Model file for the job. Use its own axes, mm. Round coordinates to 2 decimals unless told otherwise and drop trailing zeros. Order: outer loops, then holes, each group sorted by start corner. A loop starts at its lowest first (then second) coordinate and runs counter-clockwise, first axis right, second up. Notation, with made-up numbers: (43, -11) -> (89, -11) arc R13 ccw to (89, -1) -> close; hole circle Ø7 at (5, 34). An arc over 180 degrees is marked (long way). Put each result on its own line as item: value. Start each with the question number.
Q1. Probe L1, parallel to X at y = 9, z = 1.5; L2, parallel to Y at x = -11, z = 0.75 (3 decimals); L3, parallel to Y at x = 26, z = 4 (3 decimals). List the from-to ranges inside material, lowest first.
Q2. Flat gauge pins, fed straight in: P1, Ø1.9, axis at x = -16, z = 2, coming from the -Y side (3 decimals); P2, Ø4, axis at x = 24.61, y = 66.68, coming from the +Z side. Where does each tip first touch, or does it go through?
Q3. Cut at C-C, the plane x = -59.5. List the corners of the cut face in (y, z).
Q4. Cut at A-A, the plane z = 1.25. List the corners of the cut face in (x, y) (3 decimals), and give its area (3 significant figures).
Q5. Cut at B-B, the plane x = -9. List the corners of the cut face in (y, z) (3 decimals).
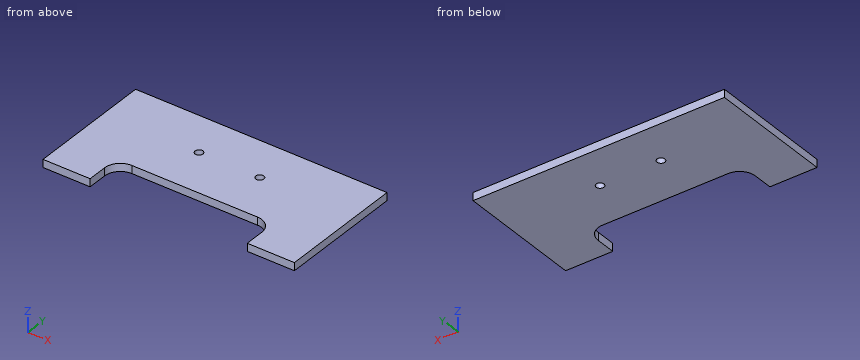
from build123d import *

# Parameters (mm, degrees)
F0_R     = 3.175
F1_DEPTH = 6.35
F2_R     = 12.7


with BuildPart() as f1:
    # F0 (on Top) → F1 (new body)
    with BuildSketch(Plane.XY):
        Polygon((0, 101.6), (-101.6, 101.6), (-101.6, 0), (-63.5, 0), (-63.5, 28.575), (0, 28.575), align=None)
        with Locations((-24.60625, 66.675)):
            Circle(F0_R, mode=Mode.SUBTRACT)
        Polygon((101.6, 101.6), (0, 101.6), (0, 28.575), (63.5, 28.575), (63.5, 0), (101.6, 0), align=None)
        with Locations((24.60625, 66.675)):
            Circle(F0_R, mode=Mode.SUBTRACT)
    extrude(amount=F1_DEPTH)

    # F2
    f2_edges = [f1.edges().sort_by_distance(p)[0] for p in [
        (-63.5, 28.575, 3.175),
        (63.5, 28.575, 3.175),
    ]]
    fillet(f2_edges, radius=F2_R)


solid = f1.part
Ans:
1. L1: x = -101.6 to -63.5, 63.5 to 101.6
1. L2: y = 28.575 to 101.6
1. L3: y = 28.575 to 63.822, 69.528 to 101.6
2. P1: stops at y = 28.575
2. P2: passes through
3. outline: (25.13, 0) -> (101.6, 0) -> (101.6, 6.35) -> (25.13, 6.35) -> close
4. outline: (-101.6, 0) -> (-63.5, 0) -> (-63.5, 15.875) arc R12.7 cw to (-50.8, 28.575) -> (50.8, 28.575) arc R12.7 cw to (63.5, 15.875) -> (63.5, 0) -> (101.6, 0) -> (101.6, 101.6) -> (-101.6, 101.6) -> close; hole circle Ø6.35 at (-24.606, 66.675); hole circle Ø6.35 at (24.606, 66.675)
4. area: 17,000 mm^2
5. outline: (28.575, 0) -> (101.6, 0) -> (101.6, 6.35) -> (28.575, 6.35) -> close
